from build123d import *

# Parameters (mm, degrees)
F1_DEPTH = 7.62
F2_R     = 38.5887386993
F2_R_2   = 31.2378777005
F3_DEPTH = 50.8
F4_W     = 40.311823599
F4_H     = 35.9383700415
F5_DEPTH = 5.334
F7_DEPTH = 44.6695281482


with BuildPart() as f1:
    # F0 (on Front) → F1 (new body)
    with BuildSketch(Plane.XZ):
        with BuildLine():
            Line((39.3345281482, -13.8564798981), (39.3345281482, 42.7613966167))
            Line((39.3345281482, 42.7613966167), (-39.3345281482, 42.7613966167))
            Line((-39.3345281482, 42.7613966167), (-39.3345281482, -13.8564798981))
            Line((-39.3345281482, -13.8564798981), (-39.3345281482, -42.7613966167))
            Line((-39.3345281482, -42.7613966167), (-39.1348331809, -42.7613966167))
            ThreePointArc((-39.1348331809, -42.7613966167), (0, -3.6265634358), (39.1348331809, -42.7613966167))
            Line((39.1348331809, -42.7613966167), (39.3345281482, -42.7613966167))
            Line((39.3345281482, -42.7613966167), (39.3345281482, -13.8564798981))
        make_face()
        with BuildLine():
            ThreePointArc((-39.1348331809, -42.7613966167), (0, -81.8962297976), (39.1348331809, -42.7613966167))
            Line((39.1348331809, -42.7613966167), (31.2378777005, -42.7613966167))
            ThreePointArc((31.2378777005, -42.7613966167), (0, -73.9992743172), (-31.2378777005, -42.7613966167))
            Line((-31.2378777005, -42.7613966167), (-39.1348331809, -42.7613966167))
        make_face()
        with BuildLine():
            Line((31.2378777005, -42.7613966167), (39.1348331809, -42.7613966167))
            ThreePointArc((39.1348331809, -42.7613966167), (0, -3.6265634358), (-39.1348331809, -42.7613966167))
            Line((-39.1348331809, -42.7613966167), (-31.2378777005, -42.7613966167))
            ThreePointArc((-31.2378777005, -42.7613966167), (0, -11.5235189162), (31.2378777005, -42.7613966167))
        make_face()
    extrude(amount=F1_DEPTH)

    # F2 (on face) → F3 (join)
    with BuildSketch(Plane.XZ.offset(7.62)):
        with Locations((0, -42.7613966167)):
            Circle(F2_R)
        with Locations((0, -42.7613966167)):
            Circle(F2_R_2, mode=Mode.SUBTRACT)
    extrude(amount=F3_DEPTH)

    # F4 (on Right) → F5 (join, symmetric)
    with BuildSketch(Plane.YZ):
        with Locations((-28.3323661424, 13.6949443258)):
            Rectangle(F4_W, F4_H)
    extrude(amount=F5_DEPTH, both=True)

    # F6 (on face) → F7 (cut, through all)
    with BuildSketch(Plane.YZ.offset(5.334)):
        Polygon((-48.4882779419, 31.6641293466), (-48.4882779419, -4.2742406949), (-8.1764543429, 31.6641293466), align=None)
    extrude(amount=-F7_DEPTH, mode=Mode.SUBTRACT)


solid = f1.part
Build history of the part. All positions in model axes, mm. A direction names the side the tool comes from. Coordinates: 2 decimals unless noted, no trailing zeros. Order: outer loops, then holes, each group sorted by start corner. A loop starts at its lowest first (then second) coordinate and runs counter-clockwise, first axis right, second up. Notation, with made-up numbers: M -13.75,-2 L 23.25,-2 A6 ccw 23.25,7 Z; hole C 35,8.5 d2. An arc over 180 degrees is marked long. One line per question, with ' | ' between items. Start each with the question number.
Q1. Saw through at B-B (z = 1). List the corners of the cut face in (x, y).
Q2. 3-axis set-ups, long thin cutter, end or side, ignore diameter. For faces 1 (the face through (-5.334, -20, 6)), 2 (the face through (-3.04, -58.42, -74.02)): which of +Z, -Z, +X, -X, +Y, -Y reach the whole face in a straight line?
Q3. Saw through at A-A (x = -23.5). List the corners of the cut face in (y, z), then the cut area to 3 significant figures.
Q4. Saw through at D-D (x = 0). List the corners of the cut face in (y, z).
Q5. Saw through at C-C (y = -34.5). List the corners of the cut face in (x, z), then the cut area to 3 significant figures.
Q6. Flat gauge pins, fed straight in: pin 1 Ø3 at (y, z) = (-30, -56.5) entering from -X; pin 2 Ø2 at (x, z) = (-29.5, -38) entering from -Y; pin 3 Ø4 at (y, z) = (-33, -11.5) entering from +X; pin 4 Ø10 at (x, y) = (30.5, -49) entering from +Z. Where does each tip first touch, or does it go through?
Q7. Two-plate mould, pull along Y, no slides. Class faces 3 (the face through (0, -8.176, 13)), 4 (the face through (5.334, -20, 6)), 5 (the face through (-1, 0, -5)): +Y half, -Y half, draft (parallel to the pull), parting line (faces both ways), or undercut.
Q8. Probe L1, parallel to Z at x = 0, y = -3; L2, parallel to X at y = -15.5, z = -42; L3, parallel to X at y = -11.5, z = -63.5. List the from-to ranges inside material, lowest first. Write a range as from..to.
Check values:
1) outline: M -39.33,-7.62 L 39.33,-7.62 L 39.33,0 L -39.33,0 Z; M -5.33,-42.57 L 5.33,-42.57 L 5.33,-8.18 L -5.33,-8.18 Z
2) face 1: +Z, -X, -Y | face 2: +Z, -Z, +X, -X, -Y
3) outline: M -58.42,-73.37 L -7.62,-73.37 L -7.62,-74.05 L 0,-74.05 L 0,-63.34 L -58.42,-63.34 Z; M -58.42,-22.18 L 0,-22.18 L 0,42.76 L -7.62,42.76 L -7.62,-12.15 L -58.42,-12.15 Z | area: 1,600 mm2
4) outline: M -58.42,-81.35 L -7.62,-81.35 L -7.62,-81.9 L 0,-81.9 L 0,-74 L -58.42,-74 Z; M -58.42,-11.52 L 0,-11.52 L 0,42.76 L -7.62,42.76 L -7.62,-4.17 L -8.18,-4.17 L -8.18,31.66 L -48.49,-4.27 L -48.49,-4.17 L -58.42,-4.17 Z
5) outline: M -5.33,-4.27 L -2.8,-4.27 A38.59 ccw long 2.8,-4.27 L 5.33,-4.27 L 5.33,8.2 L -5.33,8.2 Z; hole C 0,-42.76 d62.48 | area: 1,750 mm2
6) pin 1: stops at x = -36.6 | pin 2: passes through | pin 3: stops at x = 25.16 | pin 4: stops at z = -13.8
7) face 3: undercut | face 4: draft | face 5: +Y half
8) L1: z = -81.9..-74, -11.52..42.76 | L2: x = -38.58..-31.23, 31.23..38.58 | L3: x = -32.54..-23.36, 23.36..32.54
